The model under review builds one solid part; all positions refer to its coordinate system, in mm. Coordinates: 2 decimals unless noted, no trailing zeros. Write each loop counter-clockwise with the first axis right and the second up, starting at its lowest first coordinate (ties: lowest second). Pieces come first, ordered by that corner, then holes. Notation, with made-up numbers: M -36.5,58 L 14.5,58 A24 ccw 14.5,69 Z; hole C 3.25,-37 d1. An arc over 180 degrees is marked long. Answer as CSV lines item,"result". Start each with the question number.
from build123d import *

# Parameters (mm, degrees)
SKETCH1_R                       = 12.5
BOSS_EXTRUDE1_DEPTH             = 75
BOSS_EXTRUDE2_REACH             = 161.315
SKETCH2_R                       = 50
BOSS_EXTRUDE2_DIRECTION_2_REACH = 161.315
CHAMFER1_SIZE                   = 7.5


with BuildPart() as part:
    # Sketch1 → Boss-Extrude1 (new, symmetric)
    with BuildSketch(Plane(origin=(0, 0, 0), x_dir=(0, 0, -1), z_dir=(1, 0, 0))):
        with BuildLine():
            Line((-87.5, 0), (-87.5, 110))
            Line((-87.5, 110), (87.5, 110))
            Line((87.5, 110), (87.5, 0))
            ThreePointArc((87.5, 0), (0, -87.5), (-87.5, 0))
        make_face()
        Circle(SKETCH1_R, mode=Mode.SUBTRACT)
    extrude(amount=BOSS_EXTRUDE1_DEPTH, both=True)

    # Boss-Extrude2: up to this face of the body (flat: up to its plane)
    boss_extrude2_end = Plane(part.part.faces().sort_by_distance((0, 55, 87.5))[0])
    # Sketch2 → Boss-Extrude2 (add, up to the picked face)
    with BuildSketch(Plane.XY, mode=Mode.PRIVATE) as boss_extrude2_sk1:
        with BuildLine():
            Line((-75, 160), (-75, 85))
            Line((-75, 85), (75, 85))
            Line((75, 85), (75, 160))
            ThreePointArc((75, 160), (0, 235), (-75, 160))
        make_face()
        with Locations(Location((0, 160, 0), (0, 0, 180))):
            Circle(SKETCH2_R, mode=Mode.SUBTRACT)
    boss_extrude2_tool1 = split(extrude(boss_extrude2_sk1.sketch, amount=BOSS_EXTRUDE2_REACH, mode=Mode.PRIVATE), bisect_by=boss_extrude2_end, keep=Keep.BOTH, mode=Mode.PRIVATE)
    add(boss_extrude2_tool1.solids().sort_by(Axis((-72.87868, 122.5, 0), (0, 0, 1)))[0])

    # Boss-Extrude2 direction 2: up to this face of the body (flat: up to its plane)
    boss_extrude2_direction_2_end = Plane(part.part.faces().sort_by_distance((0, 55, -87.5))[0])
    # Sketch2 → Boss-Extrude2 direction 2 (add, up to the picked face)
    with BuildSketch(Plane.XY, mode=Mode.PRIVATE) as boss_extrude2_direction_2_sk1:
        with BuildLine():
            Line((-75, 160), (-75, 85))
            Line((-75, 85), (75, 85))
            Line((75, 85), (75, 160))
            ThreePointArc((75, 160), (0, 235), (-75, 160))
        make_face()
        with Locations(Location((0, 160, 0), (0, 0, 180))):
            Circle(SKETCH2_R, mode=Mode.SUBTRACT)
    boss_extrude2_direction_2_tool1 = split(extrude(boss_extrude2_direction_2_sk1.sketch, amount=-BOSS_EXTRUDE2_DIRECTION_2_REACH, mode=Mode.PRIVATE), bisect_by=boss_extrude2_direction_2_end, keep=Keep.BOTH, mode=Mode.PRIVATE)
    add(boss_extrude2_direction_2_tool1.solids().sort_by(Axis((-72.87868, 122.5, 0), (0, 0, -1)))[0])

    # Chamfer1
    chamfer1_edges = [part.edges().sort_by_distance(p)[0] for p in [
        (75, 80, 87.5),
        (0, 235, -87.5),
        (0, 235, 87.5),
        (75, -87.5, 0),
        (-75, 80, 87.5),
        (-75, 80, -87.5),
        (-75, -87.5, 0),
        (75, 80, -87.5),
    ]]
    chamfer(chamfer1_edges, length=CHAMFER1_SIZE)


solid = part.part
1) To check wall thickness, follow line 1 (X direction, y = 160, z = 14); line 2 (Y direction, x = -1, z = -6); line 3 (Y direction, x = -13, z = 61). State the ranges of each line that lie inside material, in increasing order. Write a range as [from, to].
2) Take a section at B-B on z = 0. Give the boundary of the cut face in (x, y), and give its area (3 significant figures).
3) Clearance check with flat-ended pins moving along their axes: pin 1 Ø15 at (y, z) = (0, 0) entering from +X; pin 2 Ø10 at (y, z) = (174.5, -32.5) entering from +X; pin 3 Ø4 at (x, y) = (56, -48.5) entering from +Z; pin 4 Ø2 at (x, z) = (44.5, -1) entering from +Y. State where each tip first meets the part, or that it passes through.
4) Take a section at A-A on x = 0. Give the boundary of the cut face in (y, z).
5) Take a section at D-D on y = 7. Give the boundary of the cut face in (x, z).
6) Mouldability with a two-part tool opening along Y and no side actions: class faces 1 (the conical face through (1.492, 227.848, 87.136)), 2 (the cylindrical face through (10.84, 208.81, -1.22)), 3 (the flat face through (71, 79, 84)), 4 (the cylindrical face through (-1.05, 3.755, -11.923)) as +Y half, -Y half, draft (parallel to the pull), parting line (faces both ways), or undercut.
7) Take a section at C-C on y = 139. Give the boundary of the cut face in (x, z).
Results:
1,line 1,"x = [-75, -50], [50, 75]"
1,line 2,"y = [-87.29, -10.97], [10.97, 110.01], [209.99, 234.99]"
1,line 3,"y = [-62.73, 111.72], [208.28, 233.86]"
2,outline,"M -75,-80 L -67.5,-87.5 L 67.5,-87.5 L 75,-80 L 75,-12.5 L -75,-12.5 Z; M -75,12.5 L 75,12.5 L 75,160 A75 ccw -75,160 Z; hole C 0,160 d100"
2,area,"34,300 mm²"
3,pin 1,"passes through"
3,pin 2,"stops at x = 74.4"
3,pin 3,"stops at z = 74.12"
3,pin 4,"stops at y = 221.1"
4,outline,"M 0,-87.5 L 110,-87.5 L 110,87.5 L 0,87.5 A87.5 ccw Z; M 210,-87.5 L 227.5,-87.5 L 235,-80 L 235,80 L 227.5,87.5 L 210,87.5 Z; hole C 0,0 d25"
5,outline,"M -75,-80 L -67.5,-87.5 L 67.5,-87.5 L 75,-80 L 75,-10.36 L -75,-10.36 Z; M -75,10.36 L 75,10.36 L 75,80 L 67.5,87.5 L -67.5,87.5 L -75,80 Z"
6,face 1,"+Y half"
6,face 2,"undercut"
6,face 3,"draft"
6,face 4,"undercut"
7,outline,"M -75,-80 L -67.5,-87.5 L -45.38,-87.5 L -45.38,87.5 L -67.5,87.5 L -75,80 Z; M 45.38,-87.5 L 67.5,-87.5 L 75,-80 L 75,80 L 67.5,87.5 L 45.38,87.5 Z"
